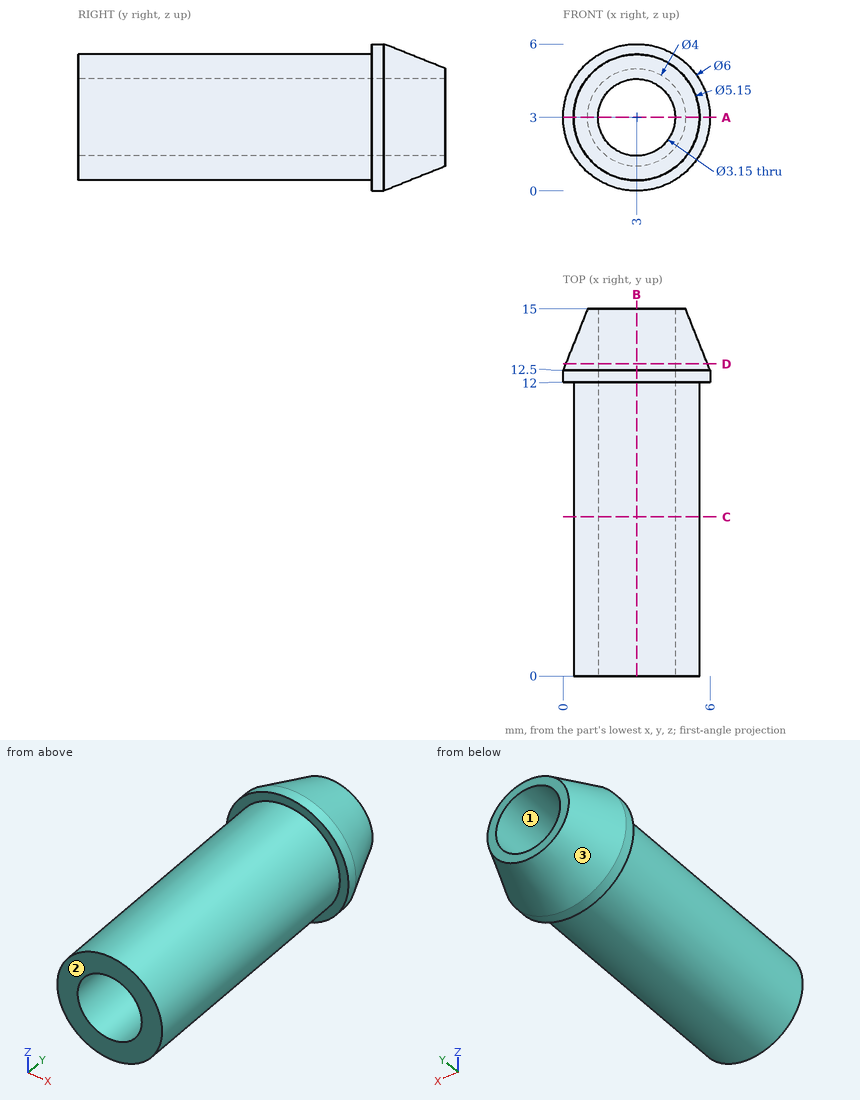
Check sheet for the drawn part. Datum: minimum x, y, z corner. Units: mm. Round coordinates to 2 decimals unless told otherwise and drop trailing zeros. Loops run counter-clockwise (first coordinate to the right, second up) from the corner with the lowest first, then second, coordinate; pieces in that order, holes last. Notation, with made-up numbers: (-25.75, 15) - (25.25, 15) arc R11 cw to (25.25, 21) - close; hole circle Ø7 at (5.5, -18). An arc over 180 degrees is marked (long way). Write item = value, one per line. Start each with the question number.
1. Depth check by flat-ended pin: pin 1 (1 mm diameter, centred on y = 6.5, z = 1, fed in from +X). Enter the tip coordinate at first touch or a pass-through.
2. Section check C-C on y = 6.5. Enter the section's corners in (x, z) (3 decimals), then the cut area to 3 significant figures.
3. Section check A-A on z = 3. Enter the section's corners in (x, y) (3 decimals).
4. Section check B-B on x = 3. Enter the section's corners in (y, z) (3 decimals).
5. Thickness scan on line 1 (Z direction, x = 3, y = 11.25) (3 decimals); line 2 (X direction, y = 7, z = 3.6). Record the ranges inside material, lowest first.
6. Section check D-D on y = 12.75. Enter the section's corners in (x, z) (3 decimals), then the cut area to 3 significant figures.
7. Mould release check, pull along Z, two halves, no side actions. Record for the marked faces 1, 2 and 3: released by +Z, released by -Z, zero draft, split by the parting line, or undercut.
Working result:
q1.pin_1 = 5.09
q2.outline = circle Ø5.15 at (3, 3); hole circle Ø3.15 at (3, 3)
q2.area = 13.0 mm^2
q3.outline = (0, 12) - (0.425, 12) - (0.425, 0) - (1.425, 0) - (1.425, 15) - (1, 15) - (0, 12.5) - close; (4.575, 0) - (5.575, 0) - (5.575, 12) - (6, 12) - (6, 12.5) - (5, 15) - (4.575, 15) - close
q4.outline = (0, 0.425) - (12, 0.425) - (12, 0) - (12.5, 0) - (15, 1) - (15, 1.425) - (0, 1.425) - close; (0, 4.575) - (15, 4.575) - (15, 5) - (12.5, 6) - (12, 6) - (12, 5.575) - (0, 5.575) - close
q5.line_1 = 0.425 to 1.425, 4.575 to 5.575
q5.line_2 = 0.5 to 1.54, 4.46 to 5.5
q6.outline = circle Ø5.8 at (3, 3); hole circle Ø3.15 at (3, 3)
q6.area = 18.6 mm^2
q7.face_1 = undercut
q7.face_2 = zero draft
q7.face_3 = split by the parting line
